from build123d import *

# Parameters (mm, degrees)
F1_DEPTH = 12.7


with BuildPart() as f1:
    # F0 (on Top) → F1 (new body)
    with BuildSketch(Plane.XY):
        Polygon((-43.18, 8.798818), (-43.18, -8.798818), (-27.94, -17.597636), (-14.559409, -9.872348), (-13.380591, -9.872348), (0, -17.597636), (13.380591, -9.872348), (14.559409, -9.872348), (27.94, -17.597636), (43.18, -8.798818), (43.18, 8.798818), (27.94, 17.597636), (14.559409, 9.872348), (13.380591, 9.872348), (0, 17.597636), (-13.380591, 9.872348), (-14.559409, 9.872348), (-27.94, 17.597636), align=None)
        Polygon((-27.94, 14.664697), (-15.24, 7.332348), (-15.24, -7.332348), (-27.94, -14.664697), (-40.64, -7.332348), (-40.64, 7.332348), align=None, mode=Mode.SUBTRACT)
        Polygon((0, -14.664697), (-12.7, -7.332348), (-12.7, 7.332348), (0, 14.664697), (12.7, 7.332348), (12.7, -7.332348), align=None, mode=Mode.SUBTRACT)
        Polygon((27.94, -14.664697), (15.24, -7.332348), (15.24, 7.332348), (27.94, 14.664697), (40.64, 7.332348), (40.64, -7.332348), align=None, mode=Mode.SUBTRACT)
    extrude(amount=F1_DEPTH)


solid = f1.part
Can you work these out from the model? Positions are in its coordinate system, mm. A direction names the side the tool comes from. Round coordinates to 2 decimals unless told otherwise and drop trailing zeros. Write each loop counter-clockwise with the first axis right and the second up, starting at its lowest first coordinate (ties: lowest second). Pieces come first, ordered by that corner, then holes. Notation, with made-up numbers: (59.25, -15) -> (88.25, -15) arc R28 cw to (88.25, 21) -> close; hole circle Ø11 at (-18.5, 82.25). An arc over 180 degrees is marked (long way). Use one line per item in the form item = value. Start each with the question number.
Q1. If I drill on probe 1 along X at (y, z) = (7, 9.75); probe 2 along X at (y, z) = (-16, 2.25); probe 3 along X at (y, z) = (-13.5, 11.25), over which ranges is the centre line in solid material (lowest first)? Write a range as [from, to].
Q2. I'm going to push flat-ended pins straight in: P1, Ø4, axis at x = 27.5, z = 6.5, coming from the -Y side; P2, Ø1.3, axis at x = 14, z = 9, coming from the -Y side; P3, Ø2, axis at x = -27, y = 11.5, coming from the -Z side; P4, Ø0.9, axis at x = 14, z = 6, coming from the +Y side. Where does each tip first touch, or does it pass through?
Q3. Imagine slicing it at B-B (x = -19). Please give me the cut outline in (y, z).
Q4. Imagine slicing it at C-C (y = 11.5). Please give me the cut outline in (x, z), then the cut area to 3 significant figures.
Q5. Imagine slicing it at D-D (z = 1.75). Count the separate pieces of the cut face and the enclosed holes in it, then the cut area to 3 significant figures.
Q6. Which directions (+Z, -Z, +X, -X, +Y, -Y) give clear straight access to the entire face, cutting with the end or side of a thin tool? Please do faces 1 (the face through (21.343, 13.789, 6.261)), 2 (the face through (21.156, -13.681, 6.261)), 3 (the face through (-13, 0, 0)), 4 (the face through (35.45, -13.26, 6.26)), 5 (the face through (12.7, 0, 6)).
Q7. We'd pull the mould along Y, two halves only. Please class faces 6 (the face through (-12.7, 0, 6)), 7 (the face through (6.784, 13.681, 6.261)), 8 (the face through (6.597, -13.789, 6.261)): +Y half, -Y half, draft (parallel to the pull), parting line (faces both ways), or undercut.
Q8. Imagine slicing it at A-A (y = 3). Please give me the cut outline in (x, z), then the cut area to 3 significant figures.
Worked out:
q1.probe_1 = [-43.18, -40.64], [-15.24, -12.7], [12.7, 15.24], [40.64, 43.18]
q1.probe_2 = [-30.71, -25.17], [-2.77, 2.77], [25.17, 30.71]
q1.probe_3 = [-35.04, -29.96], [-25.92, -20.84], [-7.1, -2.02], [2.02, 7.1], [20.84, 25.92], [29.96, 35.04]
q2.P1 = -17.6
q2.P2 = -9.92
q2.P3 = through
q2.P4 = 9.87
q3.outline = (-12.44, 0) -> (-9.5, 0) -> (-9.5, 12.7) -> (-12.44, 12.7) -> close; (9.5, 0) -> (12.44, 0) -> (12.44, 12.7) -> (9.5, 12.7) -> close
q4.outline = (-38.5, 0) -> (-33.42, 0) -> (-33.42, 12.7) -> (-38.5, 12.7) -> close; (-22.46, 0) -> (-17.38, 0) -> (-17.38, 12.7) -> (-22.46, 12.7) -> close; (-10.56, 0) -> (-5.48, 0) -> (-5.48, 12.7) -> (-10.56, 12.7) -> close; (5.48, 0) -> (10.56, 0) -> (10.56, 12.7) -> (5.48, 12.7) -> close; (17.38, 0) -> (22.46, 0) -> (22.46, 12.7) -> (17.38, 12.7) -> close; (33.42, 0) -> (38.5, 0) -> (38.5, 12.7) -> (33.42, 12.7) -> close
q4.area = 387 mm^2
q5.separate_pieces = 1
q5.enclosed_holes = 3
q5.area = 645 mm^2
q6.face_1 = +Z, -Z, +Y
q6.face_2 = +Z, -Z, -Y
q6.face_3 = -Z, +X, -X, +Y, -Y
q6.face_4 = +Z, -Z, +X, -Y
q6.face_5 = +Z, -Z
q7.face_6 = undercut
q7.face_7 = +Y half
q7.face_8 = -Y half
q8.outline = (-43.18, 0) -> (-40.64, 0) -> (-40.64, 12.7) -> (-43.18, 12.7) -> close; (-15.24, 0) -> (-12.7, 0) -> (-12.7, 12.7) -> (-15.24, 12.7) -> close; (12.7, 0) -> (15.24, 0) -> (15.24, 12.7) -> (12.7, 12.7) -> close; (40.64, 0) -> (43.18, 0) -> (43.18, 12.7) -> (40.64, 12.7) -> close
q8.area = 129 mm^2
